```python
from build123d import *

# Parameters (mm, degrees)
F1_DEPTH  = 25.4
F2_R      = 6.964249989
F3_DEPTH  = 31.75
F4_R      = 5.3902000798
F5_DEPTH  = 12.7
F6_R      = 5.8449861695
F7_DEPTH  = 12.7
F9_DEPTH  = 25.4
F11_DEPTH = 25.4
F13_DEPTH = 38.1


with BuildPart() as f1:
    # F0 (on Front) → F1 (new body)
    with BuildSketch(Plane.XZ):
        Polygon((-67.6313243027, 0), (0, 0), (0, 12.7), (-16.9078324569, 12.7), (-16.9078324569, 40.5481918725), (-48.6578324569, 40.5481918725), (-48.6578324569, 12.7), (-67.6313243027, 12.7), align=None)
    extrude(amount=F1_DEPTH)

    # F2 (on face) → F3 (cut)
    with BuildSketch(Plane.YZ.offset(-16.9078324569)):
        with Locations((-12.7, 25.5351066589)):
            Circle(F2_R)
    extrude(amount=-F3_DEPTH, mode=Mode.SUBTRACT)

    # F4 (on face) → F5 (cut)
    with BuildSketch(Plane.XY.offset(12.7)):
        with Locations((-59.1080682221, -13.0062611195)):
            Circle(F4_R)
    extrude(amount=-F5_DEPTH, mode=Mode.SUBTRACT)

    # F6 (on face) → F7 (cut)
    with BuildSketch(Plane.XY.offset(12.7)):
        with Locations((-8.3569446579, -12.7)):
            Circle(F6_R)
    extrude(amount=-F7_DEPTH, mode=Mode.SUBTRACT)

    # F8 (on face) → F9 (cut)
    with BuildSketch(Plane.XY.offset(12.7)):
        with BuildLine():
            ThreePointArc((-8.4539162285, 0), (-1.19277981, -12.1537675148), (-6.1903283931, -25.4))
            Line((-6.1903283931, -25.4), (0, -25.4))
            Line((0, -25.4), (0, 0))
            Line((0, 0), (-8.4539162285, 0))
        make_face()
    extrude(amount=-F9_DEPTH, mode=Mode.SUBTRACT)

    # F10 (on face) → F11 (cut)
    with BuildSketch(Plane.XY.offset(12.7)):
        with BuildLine():
            ThreePointArc((-60.9747394919, -25.4), (-65.9330031069, -12.7), (-60.9747394919, 0))
            Line((-60.9747394919, 0), (-67.6313243027, 0))
            Line((-67.6313243027, 0), (-67.6313243027, -25.4))
            Line((-67.6313243027, -25.4), (-60.9747394919, -25.4))
        make_face()
    extrude(amount=-F11_DEPTH, mode=Mode.SUBTRACT)

    # F12 (on face) → F13 (cut)
    with BuildSketch(Plane(origin=(-48.6578324569, 0, 0), x_dir=(0, -1, 0), z_dir=(-1, 0, 0))):
        with BuildLine():
            ThreePointArc((0, 30.7968873531), (12.8080026983, 39.50517373), (25.4, 30.487369746))
            Line((25.4, 30.487369746), (25.4, 40.5481918725))
            Line((25.4, 40.5481918725), (0, 40.5481918725))
            Line((0, 40.5481918725), (0, 30.7968873531))
        make_face()
    extrude(amount=-F13_DEPTH, mode=Mode.SUBTRACT)


solid = f1.part
```
Source: CAD feature listing. Evaluate the final solid. Frame: model axes, mm. A direction names the side the tool comes from. Give positions to 0.01 mm unless a question says otherwise; leave off trailing zeros. Order: outer loops, then holes, each group sorted by start corner. A loop starts at its lowest first (then second) coordinate and runs counter-clockwise, first axis right, second up.
(1) Section query B-B (z = 28). Return the cut outline in (x, y).
(2) Section query C-C (x = -39.5). Return the cut outline in (y, z), plus the area to 3 significant figures.
(3) Section query D-D (y = -20.5). Return the cut outline in (x, z).
(4) Contact query for flat-ended pins moving along their axis: P1, Ø10, axis at y = -7.5, z = 30, coming from the -X side; P2, Ø2, axis at x = -25.5, z = 5.5, coming from the +Y side; P3, Ø14, axis at x = -61.5, y = -17, coming from the +Z side; P4, Ø12.5, axis at x = -11, y = -15, coming from the +Z side. Output: stop coordinate, or through.
(5) Access query for faces 5 (the face through (-14, -15, 12.7)), 6 (the face through (-64.493, -12.769, 6.439)), 7 (the face through (-48.658, -9.7, 32.2)). Directions: +Z, -Z, +X, -X, +Y, -Y. A direction counts if a zero-diameter tool reaches every point of the face in a straight line with its end or side. Return the directions, or none.
(6) Material intervals for line 1 along Z through (x, y) = (-35, -12.7); line 2 along X through (y, z) = (-20, 19); line 3 along Z through (x, y) = (-59, -21.25), sorted ascending.
(7) Pull-direction query (Y, two-part tool) for faces 1 (the face through (-53, -13, 12.7)), 2 (the face through (-65.93, -12.9, 6.44)), 3 (the face through (-34, -25.4, 12)), 4 (the face through (-32.561, -9.486, 19.357)); classes: +Y half, -Y half, draft (parallel to the pull), parting line (faces both ways), or undercut.
(8) Section query A-A (y = -11). Return the cut outline in (x, z).
Outcome:
1. outline: (-48.66, -25.4) - (-16.91, -25.4) - (-16.91, -19.21) - (-48.66, -19.21) - close; (-48.66, -6.19) - (-16.91, -6.19) - (-16.91, 0) - (-48.66, 0) - close
2. outline: (-25.4, 0) - (0, 0) - (0, 30.8) arc R13.53 ccw to (-25.4, 30.49) - close; hole circle Ø13.93 at (-12.7, 25.54)
2. area: 790 mm2
3. outline: (-64.23, 0) - (-2.66, 0) - (-2.66, 12.7) - (-16.91, 12.7) - (-16.91, 36.99) - (-48.66, 36.99) - (-48.66, 12.7) - (-64.23, 12.7) - close
4. P1: stops at x = -48.66
4. P2: stops at y = 0
4. P3: stops at z = 12.7
4. P4: stops at z = 39.5
5. face 5: +Z, +X, +Y, -Y
5. face 6: +Z, -Z
5. face 7: +Z, -X, +Y, -Y
6. line 1: z = 0 to 18.57, 32.5 to 39.51
6. line 2: x = -48.66 to -16.91
6. line 3: z = 0 to 12.7
7. face 1: draft
7. face 2: parting line
7. face 3: -Y half
7. face 4: undercut
8. outline: (-65.86, 0) - (-64.11, 0) - (-64.11, 12.7) - (-65.86, 12.7) - close; (-54.11, 0) - (-13.95, 0) - (-13.95, 12.7) - (-16.91, 12.7) - (-16.91, 18.78) - (-48.66, 18.78) - (-48.66, 12.7) - (-54.11, 12.7) - close; (-48.66, 32.29) - (-16.91, 32.29) - (-16.91, 39.41) - (-48.66, 39.41) - close; (-2.76, 0) - (-1.34, 0) - (-1.34, 12.7) - (-2.76, 12.7) - close
